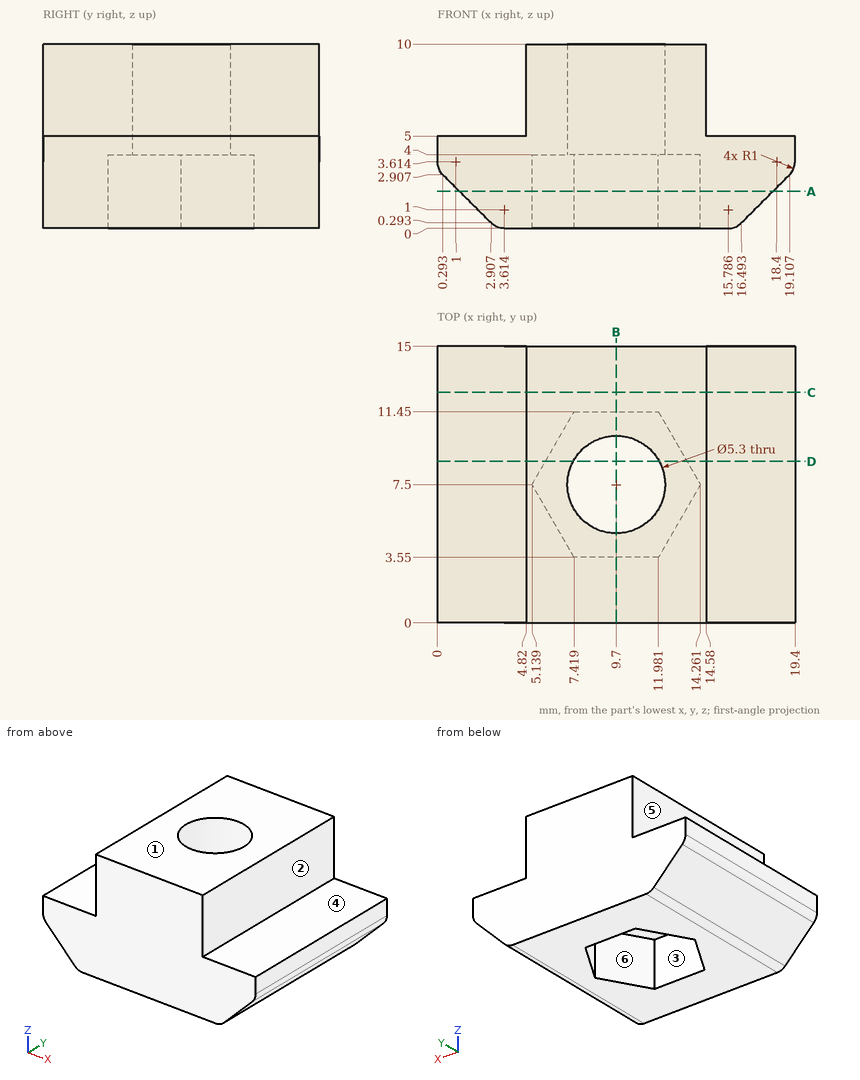
Design review of the part shown in the three views and the two pictorial views. Dimensions are in mm from the part's minimum x, y and z. A direction names the side the tool comes from. Round coordinates to 2 decimals unless told otherwise and drop trailing zeros. Loops run counter-clockwise (first coordinate to the right, second up) from the corner with the lowest first, then second, coordinate; pieces in that order, holes last. Notation, with made-up numbers: (-16.5, 61) - (8.5, 61) arc R15 cw to (8.5, 86) - close; hole circle Ø1 at (-2.5, -14.75). An arc over 180 degrees is marked (long way). Write each question's results on one line, items separated by ' | '. Start each with the question number.
Q1. Tool access review of the marked faces 4, 5 and 6: name each direction out of +Z, -Z, +X, -X, +Y, -Y from which nothing blocks a thin tool from reaching the whole face with its end or side.
Q2. Take a section at A-A on z = 2. Give the boundary of the cut face in (x, y), plus the area to 3 significant figures.
Q3. Take a section at B-B on x = 9.7. Give the boundary of the cut face in (y, z).
Q4. Draft analysis for pull direction X (two halves, no side actions). For the marked faces 1, 2 and 3, state which applies: pulls with the +X half, pulls with the -X half, needs draft (parallel to the pull), parting line crosses it, or undercut.
Q5. Take a section at D-D on y = 8.75. Give the boundary of the cut face in (x, z) (1 decimal).
Q6. Take a section at C-C on y = 12.5. Give the boundary of the cut face in (x, z) (1 decimal).
Q7. Insertion check: P1, Ø1, axis at y = 2, z = 7, coming from the +X side; P2, Ø2.5, axis at y = 5.5, z = 6.5, coming from the -X side; P3, Ø2.5, axis at x = 3.5, y = 5, coming from the +Z side. Each pin has a flat end and moves straight along its axis. Give the tip position at first contact, or say it passes through.
Q8. Wall thickness on line 1 along Y through (x, z) = (9.7, 5.35); line 2 along Y through (x, z) = (10, 0.75); line 3 along X through (y, z) = (5.5, 1) (1 decimal): over which ranges is each line inside the solid? List them lowest first. Write a range as [from, to].
Data:
1) face 4: +Z, +X, +Y, -Y | face 5: +Z, -X, +Y, -Y | face 6: -Z
2) outline: (1.2, 0) - (18.2, 0) - (18.2, 15) - (1.2, 15) - close; hole (5.14, 7.5) - (7.42, 3.55) - (11.98, 3.55) - (14.26, 7.5) - (11.98, 11.45) - (7.42, 11.45) - close | area: 201 mm²
3) outline: (0, 0) - (3.55, 0) - (3.55, 4) - (4.85, 4) - (4.85, 10) - (0, 10) - close; (10.15, 4) - (11.45, 4) - (11.45, 0) - (15, 0) - (15, 10) - (10.15, 10) - close
4) face 1: needs draft | face 2: pulls with the +X half | face 3: undercut
5) outline: (0, 3.6) arc R1 ccw to (0.3, 2.9) - (2.9, 0.3) arc R1 ccw to (3.6, 0) - (5.9, 0) - (5.9, 4) - (7.4, 4) - (7.4, 10) - (4.8, 10) - (4.8, 5) - (0, 5) - close; (12, 4) - (13.5, 4) - (13.5, 0) - (15.8, 0) arc R1 ccw to (16.5, 0.3) - (19.1, 2.9) arc R1 ccw to (19.4, 3.6) - (19.4, 5) - (14.6, 5) - (14.6, 10) - (12, 10) - close
6) outline: (0, 3.6) arc R1 ccw to (0.3, 2.9) - (2.9, 0.3) arc R1 ccw to (3.6, 0) - (15.8, 0) arc R1 ccw to (16.5, 0.3) - (19.1, 2.9) arc R1 ccw to (19.4, 3.6) - (19.4, 5) - (14.6, 5) - (14.6, 10) - (4.8, 10) - (4.8, 5) - (0, 5) - close
7) P1: stops at x = 14.58 | P2: stops at x = 4.82 | P3: stops at z = 5
8) line 1: y = [0, 4.85], [10.15, 15] | line 2: y = [0, 3.55], [11.45, 15] | line 3: x = [2.2, 6.3], [13.1, 17.2]
